```python
from build123d import *

# Parameters (mm, degrees)
EXTRUDE_1_DEPTH     = 1
CUT_EXTRUDE_1_DEPTH = 52.40107317


with BuildPart() as part:
    # 草图1 → 凸台-拉伸1 (new body)
    with BuildSketch(Plane.XY):
        Polygon((-32, 0), (32, 0), (8.783121635, 40.212812921), (0, 25), (-8.783121635, 40.212812921), align=None)
    extrude(amount=EXTRUDE_1_DEPTH)

    # 草图2 → 切除-拉伸1 (cut, through all)
    with BuildSketch(Plane.XY.offset(1)):
        Polygon((-8.783121635, 25), (-10.515172443, 22), (-8.783121635, 22), align=None)
        Polygon((-11.283121635, 17.669872981), (-11.283121635, 20.669872981), (-13.015172443, 17.669872981), align=None)
        Polygon((-13.783121635, 13.339745962), (-13.783121635, 16.339745962), (-15.515172443, 13.339745962), align=None)
        Polygon((-16.283121635, 9.009618943), (-16.283121635, 12.009618943), (-18.015172443, 9.009618943), align=None)
        Polygon((-18.783121635, 4.679491924), (-18.783121635, 7.679491924), (-20.515172443, 4.679491924), align=None)
        Polygon((-21.283121635, 0.349364905), (-21.283121635, 3.349364905), (-23.015172443, 0.349364905), align=None)
        Polygon((23.015172443, 0.349364905), (21.283121635, 0.349364905), (21.283121635, 3.349364905), align=None)
        Polygon((20.515172443, 4.679491924), (18.783121635, 4.679491924), (18.783121635, 7.679491924), align=None)
        Polygon((18.015172443, 9.009618943), (16.283121635, 9.009618943), (16.283121635, 12.009618943), align=None)
        Polygon((15.515172443, 13.339745962), (13.783121635, 13.339745962), (13.783121635, 16.339745962), align=None)
        Polygon((13.015172443, 17.669872981), (11.283121635, 17.669872981), (11.283121635, 20.669872981), align=None)
        Polygon((10.515172443, 22), (8.783121635, 22), (8.783121635, 25), align=None)
    extrude(amount=-CUT_EXTRUDE_1_DEPTH, mode=Mode.SUBTRACT)


solid = part.part
```
Input: part model. Units: mm. Frame: model coordinates. A direction names the side the tool comes from. Coordinates: 2 decimals unless noted, no trailing zeros. Write each loop counter-clockwise with the first axis right and the second up, starting at its lowest first coordinate (ties: lowest second). Pieces come first, ordered by that corner, then holes. Notation, with made-up numbers: M 74,79.5 L 115,79.5 A26 ccw 115,108.5 Z; hole C -9,-31.75 d11. An arc over 180 degrees is marked long. Use one line per item in the form item = value.
Q1. Section A-A (y = 33). Return loops of the section in (x, z).
Answer below:
outline = M -12.95,0 L -4.62,0 L -4.62,1 L -12.95,1 Z; M 4.62,0 L 12.95,0 L 12.95,1 L 4.62,1 Z
Q2. Material intervals for probe 1 along X at (y, z) = (24.5, 0.95); probe 2 along X at (y, z) = (2.5, 0.9); probe 3 along X at (y, z) = (28, 0.7), sorted ascending. Write a range as from..to.
Answer below:
probe_1 = -17.85..-9.07, -8.78..8.78, 9.07..17.85
probe_2 = -30.56..-21.77, -21.28..21.28, 21.77..30.56
probe_3 = -15.83..-1.73, 1.73..15.83
Q3. Section B-B (z = 0.45). Count the separate pieces of the cut face and the enclosed holes in it, plus the area to 3 significant figures.
Answer below:
separate_pieces = 1
enclosed_holes = 12
area = 1,480 mm²
Q4. Section C-C (y = 27). Return loops of the section in (x, z).
Answer below:
outline = M -16.41,0 L -1.15,0 L -1.15,1 L -16.41,1 Z; M 1.15,0 L 16.41,0 L 16.41,1 L 1.15,1 Z
Q5. First-contact query: pin 1 (0.5 mm diameter, centred on y = 5.5, z = 0.5, fed in from -X); pin 2 (0.5 mm diameter, centred on x = -12, z = 0.5, fed in from +Y); pin 3 (0.5 mm diameter, centred on x = 17.5, z = 0.5, fed in from +Y). Flat tips, straight axial feed; report the tip coordinate or a pass-through.
Answer below:
pin_1 = -28.97
pin_2 = 35.07
pin_3 = 25.55
Q6. Section D-D (x = 8). Return loops of the section in (y, z), plus the area to 3 significant figures.
Answer below:
outline = M 0,0 L 38.86,0 L 38.86,1 L 0,1 Z
area = 38.9 mm²
Q7. Draft query along X for faces 3 (the face through (12.137, 19.191, 0.507)), 4 (the face through (20.554, 19.825, 0.493)), 5 (the face through (14.637, 14.861, 0.507)), 6 (the face through (0, 16, 0)). Return one class per face: released by +X, released by -X, zero draft, split by the parting line, or undercut.
Answer below:
face_3 = undercut
face_4 = released by +X
face_5 = undercut
face_6 = zero draft
Q8. Set-up query: faces 1 (the face through (-4.33, 32.5, 0.49)), 2 (the face through (0, 16, 1)). Return all of +Z, -Z, +X, -X, +Y, -Y with unobstructed straight access to the full face (end or side cutting, diameter ignored); none if empty.
Answer below:
face_1 = +Z, -Z, +Y
face_2 = +Z, +X, -X, +Y, -Y
